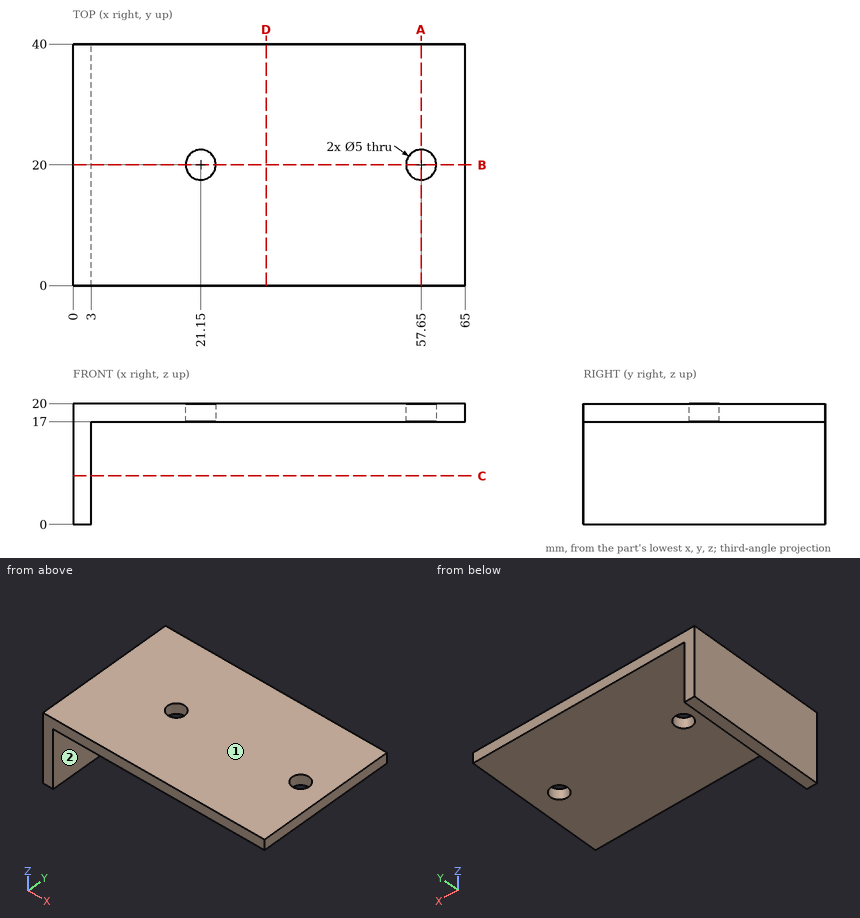
Design review of the part shown in the three views and the two pictorial views. Dimensions are in mm from the part's minimum x, y and z. A direction names the side the tool comes from. Round coordinates to 2 decimals unless told otherwise and drop trailing zeros. Loops run counter-clockwise (first coordinate to the right, second up) from the corner with the lowest first, then second, coordinate; pieces in that order, holes last.
Q1. Machinability: for the marked faces 1 and 2, which of the approach directions +Z, -Z, +X, -X, +Y, -Y give a long, thin tool a straight path to every point of the face, cutting with its end or side? Answer none if there is none.
Result sheet:
face 1: +Z, +X, -X, +Y, -Y
face 2: -Z, +X, +Y, -Y
Q2. Add section B-B on y = 20. Write out the cut boundary in (x, z), plus the area to 3 significant figures.
Result sheet:
outline: (0, 0) - (3, 0) - (3, 17) - (18.65, 17) - (18.65, 20) - (0, 20) - close; (23.65, 17) - (55.15, 17) - (55.15, 20) - (23.65, 20) - close; (60.15, 17) - (65, 17) - (65, 20) - (60.15, 20) - close
area: 216 mm2
Q3. To check wall thickness, follow line 1 along Y through (x, z) = (21.15, 17.7); line 2 along Z through (x, y) = (62.5, 17.5); line 3 along X through (y, z) = (10, 2.25). State the ranges of each line that lie inside material, in increasing order.
Result sheet:
line 1: y = 0 to 17.5, 22.5 to 40
line 2: z = 17 to 20
line 3: x = 0 to 3
Q4. Add section D-D on x = 32. Write out the cut boundary in (y, z).
Result sheet:
outline: (0, 17) - (40, 17) - (40, 20) - (0, 20) - close
Q5. Add section C-C on z = 8. Write out the cut boundary in (x, y), plus the area to 3 significant figures.
Result sheet:
outline: (0, 0) - (3, 0) - (3, 40) - (0, 40) - close
area: 120 mm2
Q6. Insertion check: pin 1 Ø5 at (y, z) = (31.5, 16) entering from +X; pin 2 Ø12 at (x, y) = (23, 29) entering from -Z; pin 3 Ø3 at (y, z) = (27.5, 14.5) entering from +X. Each pin has a flat end and moves straight along its axis. Give the tip position at first contact, or say it passes through.
Result sheet:
pin 1: stops at x = 65
pin 2: stops at z = 17
pin 3: stops at x = 3
Q7. Add section A-A on x = 57.65. Write out the cut boundary in (y, z), plus the area to 3 significant figures.
Result sheet:
outline: (0, 17) - (17.5, 17) - (17.5, 20) - (0, 20) - close; (22.5, 17) - (40, 17) - (40, 20) - (22.5, 20) - close
area: 105 mm2
